Build history of the part. All positions in model axes, mm. Face numbers are marked on the shaded views. A direction names the side the tool comes from. Coordinates: 2 decimals unless noted, no trailing zeros. Loops run counter-clockwise (first coordinate to the right, second up) from the corner with the lowest first, then second, coordinate; pieces in that order, holes last.
(1) Slice it at A-A (z = 10). Give the cut face in (x, y).
(2) Wall check: L1, parallel to Y at x = 0, z = 7; L2, parallel to Y at x = 0, z = 9; L3, parallel to Z at x = 28, y = -3.5. Give the ranges that are in metal, low to high.
(3) Two-plate mould, pull along Y, no slides. Class the marked faces 1, 2 and 3: pulls with the +Y half, pulls with the -Y half, needs draft (parallel to the pull), parting line crosses it, or undercut.
(4) Tool access for the marked faces 4 and 5: list every direction of +Z, -Z, +X, -X, +Y, -Y with a clear straight run to the whole face (end or side of a thin tool).
(5) Slice it at B-B (z = 24.5). Give the cut face in (x, y), and give its area (3 significant figures).
(6) Flat gauge pins, fed straight in: P1, Ø6, axis at x = -23.5, z = 8.5, coming from the -Y side; P2, Ø1, axis at y = -12.5, z = 41.5, coming from the +X side; P3, Ø1.5, axis at x = -19, z = 20, coming from the +Y side. Where does each tip first touch, or does it go through?
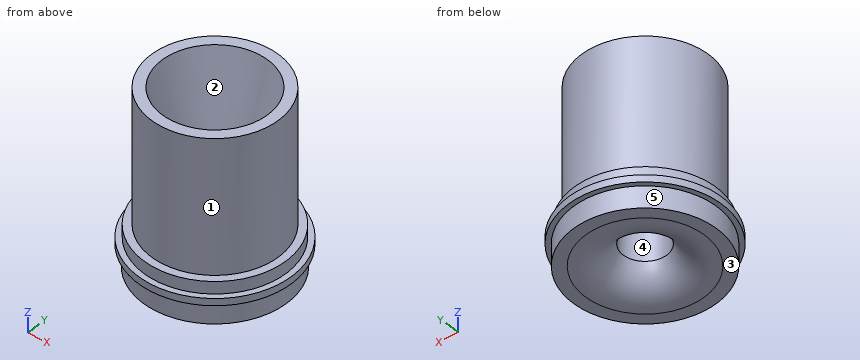
from build123d import *


with BuildPart() as part:
    # Sketch1 → Revolve4 (revolve)
    with BuildSketch(Plane(origin=(0, 0, 0), x_dir=(1, 0, 0), z_dir=(0, 1, 0)), mode=Mode.PRIVATE) as revolve4_sk:
        with BuildLine():
            add(Edge.make_bspline(
                [(9.779, 0), (14.416661489, 10.52798938), (26.83, 9.72)],
                knots=[0, 0, 0, 1, 1, 1], degree=2))
            Line((26.83, 9.72), (32.33, 9.72))
            Line((32.33, 9.72), (32.33, 0))
            Line((32.33, 0), (34.5, 0))
            Line((34.5, 0), (34.5, -3.170406434))
            Line((34.5, -3.170406434), (32, -3.170406434))
            Line((32, -3.170406434), (32, -8.670406434))
            Line((32, -8.670406434), (28.6, -8.670406434))
            Line((28.6, -8.670406434), (28.6, -68.670406434))
            Line((28.6, -68.670406434), (23.8, -68.670406434))
            Line((23.8, -68.670406434), (9.779, -13.6226))
            Line((9.779, -13.6226), (9.779, -8.8474))
            Line((9.779, -8.8474), (9.779, 0))
        make_face()
    revolve(revolve4_sk.sketch.rotate(Axis((0, 0, 0), (0, 0, 1)), 180), axis=Axis((0, 0, 0), (0, 0, 1)))


solid = part.part
Response values:
1. outline: circle Ø57.2 at (0, 0); hole circle Ø19.56 at (0, 0)
2. L1: y = -32 to -9.78, 9.78 to 32
2. L2: y = -28.6 to -9.78, 9.78 to 28.6
2. L3: z = -9.72 to 68.67
3. face 1: parting line crosses it
3. face 2: undercut
3. face 3: needs draft
4. face 4: +Z, -Z
4. face 5: -Z
5. outline: circle Ø57.2 at (0, 0); hole circle Ø25.1 at (0, 0)
5. area: 2,070 mm2
6. P1: stops at y = -24.57
6. P2: stops at x = 25.96
6. P3: stops at y = 22.02
